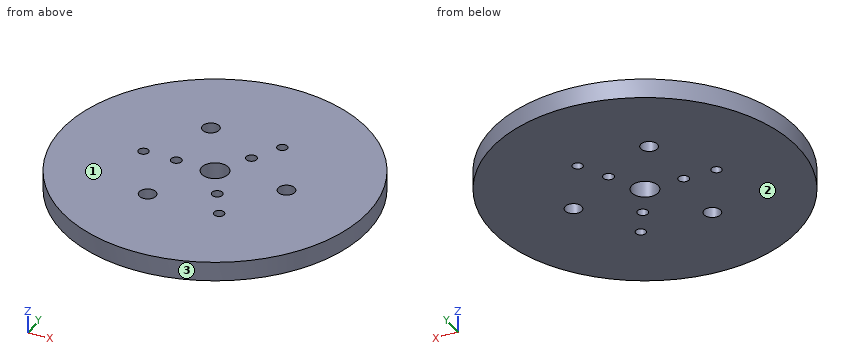
```python
from build123d import *

# Parameters (mm, degrees)
CROQUIS1_R              = 75
SALIENTE_EXTRUIR1_DEPTH = 9.53
CORTAR_EXTRUIR1_REACH   = 11.53
CROQUIS2_R              = 4.1
CORTAR_EXTRUIR2_REACH   = 11.53
CROQUIS3_R              = 6.5
CORTAR_EXTRUIR3_REACH   = 11.53
CROQUIS4_R              = 2.6
CORTAR_EXTRUIR4_REACH   = 11.53
CROQUIS5_R              = 2.5


with BuildPart() as part:
    # Croquis1 → Saliente-Extruir1 (new body)
    with BuildSketch(Plane.XY):
        Circle(CROQUIS1_R)
    extrude(amount=SALIENTE_EXTRUIR1_DEPTH)

    # Croquis2 → Cortar-Extruir1 (cut, up to next)
    with BuildSketch(Plane(origin=(0, 0, 0), x_dir=(-1, 0, 0), z_dir=(0, 0, -1)), mode=Mode.PRIVATE) as cortar_extruir1_sk1:
        with Locations((-35, 0)):
            Circle(CROQUIS2_R)
    cortar_extruir1_tool1 = extrude(cortar_extruir1_sk1.sketch, amount=-CORTAR_EXTRUIR1_REACH, mode=Mode.PRIVATE) & part.part
    add(cortar_extruir1_tool1.solids().sort_by_distance((35, 0, 0))[0], mode=Mode.SUBTRACT)
    # Croquis2 → Cortar-Extruir1 (cut, up to next)
    with BuildSketch(Plane(origin=(0, 0, 0), x_dir=(-1, 0, 0), z_dir=(0, 0, -1)), mode=Mode.PRIVATE) as cortar_extruir1_sk2:
        with Locations((17.5, 30.310889132)):
            Circle(CROQUIS2_R)
    cortar_extruir1_tool2 = extrude(cortar_extruir1_sk2.sketch, amount=-CORTAR_EXTRUIR1_REACH, mode=Mode.PRIVATE) & part.part
    add(cortar_extruir1_tool2.solids().sort_by_distance((-17.5, 30.310889, 0))[0], mode=Mode.SUBTRACT)
    # Croquis2 → Cortar-Extruir1 (cut, up to next)
    with BuildSketch(Plane(origin=(0, 0, 0), x_dir=(-1, 0, 0), z_dir=(0, 0, -1)), mode=Mode.PRIVATE) as cortar_extruir1_sk3:
        with Locations((17.5, -30.310889132)):
            Circle(CROQUIS2_R)
    cortar_extruir1_tool3 = extrude(cortar_extruir1_sk3.sketch, amount=-CORTAR_EXTRUIR1_REACH, mode=Mode.PRIVATE) & part.part
    add(cortar_extruir1_tool3.solids().sort_by_distance((-17.5, -30.310889, 0))[0], mode=Mode.SUBTRACT)

    # Croquis3 → Cortar-Extruir2 (cut, up to next)
    with BuildSketch(Plane(origin=(0, 0, 0), x_dir=(-1, 0, 0), z_dir=(0, 0, -1)), mode=Mode.PRIVATE) as cortar_extruir2_sk1:
        Circle(CROQUIS3_R)
    cortar_extruir2_tool1 = extrude(cortar_extruir2_sk1.sketch, amount=-CORTAR_EXTRUIR2_REACH, mode=Mode.PRIVATE) & part.part
    add(cortar_extruir2_tool1.solids().sort_by_distance((0, 0, 0))[0], mode=Mode.SUBTRACT)

    # Croquis4 → Cortar-Extruir3 (cut, up to next)
    with BuildSketch(Plane.XY.offset(9.53), mode=Mode.PRIVATE) as cortar_extruir3_sk1:
        with Locations((-18.937088829, 0)):
            Circle(CROQUIS4_R)
    cortar_extruir3_tool1 = extrude(cortar_extruir3_sk1.sketch, amount=-CORTAR_EXTRUIR3_REACH, mode=Mode.PRIVATE) & part.part
    add(cortar_extruir3_tool1.solids().sort_by_distance((-18.937089, 0, 9.53))[0], mode=Mode.SUBTRACT)
    # Croquis4 → Cortar-Extruir3 (cut, up to next)
    with BuildSketch(Plane.XY.offset(9.53), mode=Mode.PRIVATE) as cortar_extruir3_sk2:
        with Locations((9.468544415, 16.4)):
            Circle(CROQUIS4_R)
    cortar_extruir3_tool2 = extrude(cortar_extruir3_sk2.sketch, amount=-CORTAR_EXTRUIR3_REACH, mode=Mode.PRIVATE) & part.part
    add(cortar_extruir3_tool2.solids().sort_by_distance((9.468544, 16.4, 9.53))[0], mode=Mode.SUBTRACT)
    # Croquis4 → Cortar-Extruir3 (cut, up to next)
    with BuildSketch(Plane.XY.offset(9.53), mode=Mode.PRIVATE) as cortar_extruir3_sk3:
        with Locations((9.468544415, -16.4)):
            Circle(CROQUIS4_R)
    cortar_extruir3_tool3 = extrude(cortar_extruir3_sk3.sketch, amount=-CORTAR_EXTRUIR3_REACH, mode=Mode.PRIVATE) & part.part
    add(cortar_extruir3_tool3.solids().sort_by_distance((9.468544, -16.4, 9.53))[0], mode=Mode.SUBTRACT)

    # Croquis5 → Cortar-Extruir4 (cut, up to next)
    with BuildSketch(Plane.XY.offset(9.53), mode=Mode.PRIVATE) as cortar_extruir4_sk1:
        with Locations((-35, 0)):
            Circle(CROQUIS5_R)
    cortar_extruir4_tool1 = extrude(cortar_extruir4_sk1.sketch, amount=-CORTAR_EXTRUIR4_REACH, mode=Mode.PRIVATE) & part.part
    add(cortar_extruir4_tool1.solids().sort_by_distance((-35, 0, 9.53))[0], mode=Mode.SUBTRACT)
    # Croquis5 → Cortar-Extruir4 (cut, up to next)
    with BuildSketch(Plane.XY.offset(9.53), mode=Mode.PRIVATE) as cortar_extruir4_sk2:
        with Locations((17.5, 30.310889132)):
            Circle(CROQUIS5_R)
    cortar_extruir4_tool2 = extrude(cortar_extruir4_sk2.sketch, amount=-CORTAR_EXTRUIR4_REACH, mode=Mode.PRIVATE) & part.part
    add(cortar_extruir4_tool2.solids().sort_by_distance((17.5, 30.310889, 9.53))[0], mode=Mode.SUBTRACT)
    # Croquis5 → Cortar-Extruir4 (cut, up to next)
    with BuildSketch(Plane.XY.offset(9.53), mode=Mode.PRIVATE) as cortar_extruir4_sk3:
        with Locations((17.5, -30.310889132)):
            Circle(CROQUIS5_R)
    cortar_extruir4_tool3 = extrude(cortar_extruir4_sk3.sketch, amount=-CORTAR_EXTRUIR4_REACH, mode=Mode.PRIVATE) & part.part
    add(cortar_extruir4_tool3.solids().sort_by_distance((17.5, -30.310889, 9.53))[0], mode=Mode.SUBTRACT)


solid = part.part
```
Can you work these out from the model? Positions are in its coordinate system, mm. Face numbers are marked on the shaded views. Round coordinates to 2 decimals unless told otherwise and drop trailing zeros. Order: outer loops, then holes, each group sorted by start corner. A loop starts at its lowest first (then second) coordinate and runs counter-clockwise, first axis right, second up. Notation, with made-up numbers: (14.25, 61.5) -> (64.25, 61.5) arc R28 cw to (64.25, 87.5) -> close; hole circle Ø2 at (47.25, -38). An arc over 180 degrees is marked (long way). Return JSON: item names as keys, results as strings. Group by question number.
1. If we section it at C-C, the plane y = -16.4: Write out the boundary of the cut face in (x, z).
2. We'd pull the mould along Z, two halves only. Please class the marked faces 1, 2 and 3: released by +Z, released by -Z, zero draft, split by the parting line, or undercut.
3. I need wall thicknesses on line 1 (Y direction, x = 0, z = 7.5); line 2 (Y direction, x = -17.5, z = 7.25); line 3 (Y direction, x = 19.5, z = 2.75). Which ranges of each line are inside material? Lowest first, please. Write a range as [from, to].
4. If we section it at D-D, the plane z = 5: Count the separate pieces of the cut face and the enclosed holes in it, then the cut area to 3 significant figures.
5. If we section it at B-B, the plane x = -35: Write out the boundary of the cut face in (y, z), then the cut area to 3 significant figures.
6. Will these pins go through, and if not, where does the flat tip stop? pin 1 (3 mm diameter, centred on x = 9.47, y = 16.4, fed in from +Z); pin 2 (3 mm diameter, centred on x = -42, z = 6, fed in from +Y); pin 3 (2 mm diameter, centred on y = 4.5, z = 3, fed in from -X).
7. If we section it at A-A, the plane y = 0: Write out the boundary of the cut face in (x, z).
Output values:
{
 "1": {"outline": "(-73.18, 0) -> (6.87, 0) -> (6.87, 9.53) -> (-73.18, 9.53) -> close; (12.07, 0) -> (73.18, 0) -> (73.18, 9.53) -> (12.07, 9.53) -> close"},
 "2": {"face 1": "released by +Z", "face 2": "released by -Z", "face 3": "zero draft"},
 "3": {"line 1": "[-75, -6.5], [6.5, 75]", "line 2": "[-72.93, -34.41], [-26.21, -2.17], [2.17, 26.21], [34.41, 72.93]", "line 3": "[-72.42, -31.81], [-28.81, 28.81], [31.81, 72.42]"},
 "4": {"separate pieces": "1", "enclosed holes": "10", "area": "17,300 mm²"},
 "5": {"outline": "(-66.33, 0) -> (-2.5, 0) -> (-2.5, 9.53) -> (-66.33, 9.53) -> close; (2.5, 0) -> (66.33, 0) -> (66.33, 9.53) -> (2.5, 9.53) -> close", "area": "1,220 mm²"},
 "6": {"pin 1": "through", "pin 2": "y = 63.12", "pin 3": "x = -74.92"},
 "7": {"outline": "(-75, 0) -> (-37.5, 0) -> (-37.5, 9.53) -> (-75, 9.53) -> close; (-32.5, 0) -> (-21.54, 0) -> (-21.54, 9.53) -> (-32.5, 9.53) -> close; (-16.34, 0) -> (-6.5, 0) -> (-6.5, 9.53) -> (-16.34, 9.53) -> close; (6.5, 0) -> (30.9, 0) -> (30.9, 9.53) -> (6.5, 9.53) -> close; (39.1, 0) -> (75, 0) -> (75, 9.53) -> (39.1, 9.53) -> close"}
}
